Can you work these out from the model? Positions are in its coordinate system, mm. Face numbers are marked on the shaded views. Give positions to 0.01 mm unless a question says otherwise; leave off trailing zeros. Loops run counter-clockwise (first coordinate to the right, second up) from the corner with the lowest first, then second, coordinate; pieces in that order, holes last. Notation, with made-up numbers: (-1.75, 6) - (27.25, 6) arc R16 ccw to (27.25, 23) - close; hole circle Ø10 at (72, -22.5). An arc over 180 degrees is marked (long way). Answer as a JSON object with one key per item and string values.
Autodesk Inventor part; units mm, degrees
ref_plane "Płaszczyzna konstrukcyjna1" through (26, 12.3744, 12.3744) normal (0, 0.7071068, 0.7071068) x (-1, 0, 0)
ref_plane "Płaszczyzna konstrukcyjna2" through (26, 12.3744, -12.3744) normal (0, 0.7071068, -0.7071068) x (-1, 0, 0)
ref_plane "YZ Plane" through (0, 0, 0) normal (1, 0, 0) x (0, 1, 0)
sketch "Szkic1" plane through (0, 0, 0) normal (1, 0, 0) x (0, 1, 0)
  circle A0 centre (0, 0) radius 17.5
  dimension "d0" = 35
extrude "Wyciągnięcie proste1" add sketch "Szkic1" along normal blind 26
sketch "Szkic2" plane through (26, 0, 0) normal (1, 0, 0) x (0, 0, -1)
  point P0 (0, 0)
  point P1 (0, 0)
hole "Otwór1" at (26, 0, 0) direction (-1, 0, 0) diameter 8 end through all
sketch "Szkic3" plane through (26, 0, 0) normal (1, 0, 0) x (0, 0, -1)
  point P0 (0, 0)
  point P1 (13.5, 0)
  point P2 (0, 13.5)
  point P3 (-13.5, 0)
  point P4 (0, -13.5)
  dimension "d10" = 13.5
  dimension "d13" = 360
hole "Otwór2" at (26, 0, -13.5) at (26, 13.5, 0) at (26, 0, 13.5) at (26, -13.5, 0) direction (-1, 0, 0) diameter 3.5 depth 26 tip angle 118
sketch "Szkic4" plane through (26, 0, 0) normal (1, 0, 0) x (0, 0, -1)
  line L0 (0, 0) -> (-12.3744, 12.3744)
  line L1 (0, 0) -> (17.5, 0) construction
  line L2 (0, 0) -> (12.3744, 12.3744)
  line L3 (0, 0) -> (17.5, 0) construction
  dimension "d22" = 17.5
  dimension "d23" = 135
  dimension "d24" = 17.5
  dimension "d25" = 45
ref_plane "Płaszczyzna konstrukcyjna1" through (26, 12.3744, 12.3744) normal (0, 0.7071068, 0.7071068) x (-1, 0, 0)
ref_plane "Płaszczyzna konstrukcyjna2" through (26, 12.3744, -12.3744) normal (0, 0.7071068, -0.7071068) x (-1, 0, 0)
sketch "Szkic10" plane through (26, 12.3744, 12.3744) normal (0, 0.7071068, 0.7071068) x (-1, 0, 0)
  line L0 (26, -17.5) -> (26, 17.5)
  line L1 (0, 17.5) -> (0, -17.5)
  line L2 (26, 17.5) -> (0, 17.5)
  line L3 (26, -17.5) -> (0, -17.5)
  point P0 (26, 0)
  point P1 (13, 0)
  dimension "d54" = 13
  dimension "d55" = 26
  dimension "d56" = 35
  dimension "d57" = 17.5
hole "Otwór5" at (13, 12.3744, 12.3744) direction (0, -0.7071068, -0.7071068) diameter 4.134 end up to surface
sketch "Szkic12" plane through (26, 12.3744, -12.3744) normal (0, 0.7071068, -0.7071068) x (-1, 0, 0)
  line L0 (26, 17.5) -> (0, 17.5)
  line L1 (26, -17.5) -> (26, 17.5)
  line L2 (26, -17.5) -> (0, -17.5)
  line L3 (0, 17.5) -> (0, -17.5)
  point P0 (26, 0)
  point P1 (13, 0)
  dimension "d67" = 35
  dimension "d68" = 26
  dimension "d69" = 13
  dimension "d70" = 17.5
hole "Otwór6" at (13, 12.3744, -12.3744) direction (0, -0.7071068, 0.7071068) diameter 4.134 end up to surface
equation "\"d0\" = radius"
equation "\"d16\" = d1"
equation "\"d20\" = d1"
equation "\"d22\" = 0.5 * radius"
equation "\"d24\" = d22"
equation "\"radius\" = 35"
properties part number "piasta_kola_napedowego_fi8" material "Aluminum 6061"
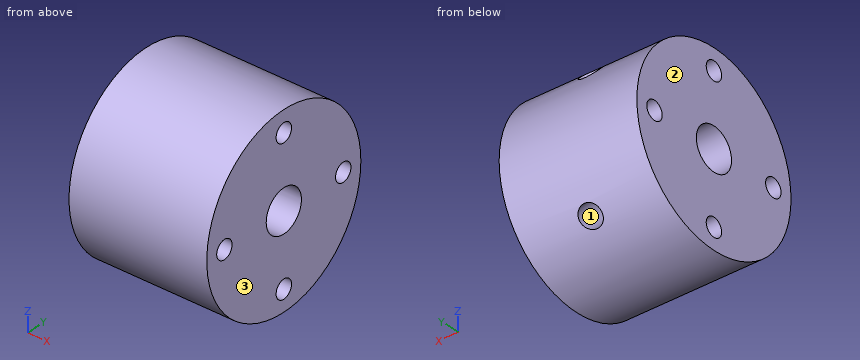
1) Imagine slicing it at B-B on x = 21.75. Write out the boundary of the cut face in (y, z).
Check sheet entries:
{"outline": "circle Ø35 at (0, 0); hole circle Ø3.5 at (-13.5, 0); hole circle Ø8 at (0, 0); hole circle Ø3.5 at (0, -13.5); hole circle Ø3.5 at (0, 13.5); hole circle Ø3.5 at (13.5, 0)"}
2) Imagine slicing it at D-D on y = -13.5. Write out the boundary of the cut face in (x, z), and give its area (3 significant figures).
Check sheet entries:
{"outline": "(0, -11.14) - (26, -11.14) - (26, -1.75) - (0, -1.75) - close; (0, 1.75) - (26, 1.75) - (26, 11.14) - (0, 11.14) - close", "area": "488 mm2"}
3) Imagine slicing it at A-A on y = 0. Write out the boundary of the cut face in (x, z).
Check sheet entries:
{"outline": "(0, -17.5) - (26, -17.5) - (26, -15.25) - (0, -15.25) - close; (0, -11.75) - (26, -11.75) - (26, -4) - (0, -4) - close; (0, 4) - (26, 4) - (26, 11.75) - (0, 11.75) - close; (0, 15.25) - (26, 15.25) - (26, 17.5) - (0, 17.5) - close"}
4) Imagine slicing it at C-C on z = 14.5. Write out the boundary of the cut face in (x, y), and give its area (3 significant figures).
Check sheet entries:
{"outline": "(0, -9.8) - (26, -9.8) - (26, -1.44) - (0, -1.44) - close; (0, 1.44) - (26, 1.44) - (26, 9.8) - (0, 9.8) - close", "area": "435 mm2"}
5) If we mould it in two halves opening along X, with no side actions, what happens to the marked faces 1, 2 and 3? For each: released by +X, released by -X, zero draft, split by the parting line, or undercut.
Check sheet entries:
{"face 1": "undercut", "face 2": "released by -X", "face 3": "released by +X"}
6) I'm going to push flat-ended pins straight in: P1, Ø4, axis at x = 20.5, z = -4.5, coming from the +Y side; P2, Ø12, axis at x = 8.5, y = 10, coming from the +Z side; P3, Ø2, axis at y = 0, z = -13.5, coming from the +X side; P4, Ø1.5, axis at x = 18.5, z = 9.5, coming from the -Y side. Where does each tip first touch, or does it pass through?
Check sheet entries:
{"P1": "y = 17.32", "P2": "z = 17.04", "P3": "through", "P4": "y = -15.16"}
7) I need wall thicknesses on L1, parallel to Z at x = 6.5, y = 0; L2, parallel to Z at x = 13.25, y = 8; L3, parallel to Y at x = 1.75, z = -0.5. Which ranges of each line are inside material? Lowest first, please.
Check sheet entries:
{"L1": "-17.5 to -15.25, -11.75 to -4, 4 to 11.75, 15.25 to 17.5", "L2": "-15.56 to -10.9, -5.1 to 5.1, 10.9 to 15.56", "L3": "-17.49 to -15.18, -11.82 to -3.97, 3.97 to 11.82, 15.18 to 17.49"}
